The model under review builds one solid part; all positions refer to its coordinate system, in mm. Face numbers are marked on the shaded views. A direction names the side the tool comes from. Give positions to 0.01 mm unless a question says otherwise; leave off trailing zeros. Order: outer loops, then holes, each group sorted by start corner. A loop starts at its lowest first (then second) coordinate and runs counter-clockwise, first axis right, second up. Notation, with made-up numbers: (87, 59) - (132, 59) arc R22 cw to (132, 92) - close; hole circle Ø3 at (7.25, -21). An arc over 180 degrees is marked (long way). Put each result on its own line as item: value.
```python
from build123d import *
from build123d.topology import SkipClean

# Parameters (mm, degrees)
SKETCH1_R           = 1
SKETCH1_R_2         = 0.9
BOSS_EXTRUDE1_DEPTH = 10
SKETCH2_R           = 1
SKETCH2_R_2         = 0.9
BOSS_EXTRUDE2_DEPTH = 5
SKETCH4_R           = 0.9
CUT_EXTRUDE2_DEPTH  = 12.224972294
SKETCH5_R           = 0.9
CUT_EXTRUDE3_DEPTH  = 15.17744702


with BuildPart() as part:
    # Sketch1 → Boss-Extrude1 (new body)
    with BuildSketch(Plane(origin=(0, 0, 0), x_dir=(1, 0, 0), z_dir=(0, 1, 0))):
        with Locations(Location((0, 0, 0), (0, 0, 270))):
            Circle(SKETCH1_R)
        with Locations(Location((0, 0, 0), (0, 0, 270))):
            Circle(SKETCH1_R_2, mode=Mode.SUBTRACT)
    extrude(amount=BOSS_EXTRUDE1_DEPTH)

    # Sketch2 → Boss-Extrude2 (add, symmetric)
    with BuildSketch(Plane(origin=(0, 0, 0), x_dir=(0, 0, -1), z_dir=(1, 0, 0))):
        with Locations((0, 5)):
            Circle(SKETCH2_R)
        with Locations(Location((0, 5, 0), (0, 0, 180))):
            Circle(SKETCH2_R_2, mode=Mode.SUBTRACT)
    extrude(amount=BOSS_EXTRUDE2_DEPTH, both=True)

    # Sketch4 → Cut-Extrude2 (cut, through all)
    with BuildSketch(Plane.XZ):
        with Locations(Location((0, 0, 0), (0, 0, 90))):
            Circle(SKETCH4_R)
    extrude(amount=-CUT_EXTRUDE2_DEPTH, mode=Mode.SUBTRACT)

    # Sketch5 → Cut-Extrude3 (cut, through all)
    with SkipClean():  # the faces are left unmerged after this step: merging them gives an invalid solid
        with BuildSketch(Plane(origin=(5, 0, 0), x_dir=(0, 0, -1), z_dir=(1, 0, 0))):
            with Locations((0, 5)):
                Circle(SKETCH5_R)
        extrude(amount=-CUT_EXTRUDE3_DEPTH, mode=Mode.SUBTRACT)


solid = part.part
```
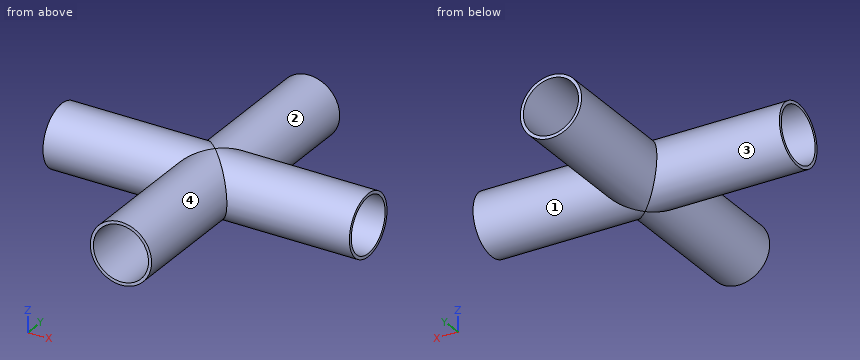
(1) The part is to be moulded in two halves that separate along Y. For the marked faces 1 and 2, say which applies: pulls with the +Y half, pulls with the -Y half, needs draft (parallel to the pull), parting line crosses it, or undercut.
The answers:
face 1: parting line crosses it
face 2: needs draft
(2) Take a section at D-D, the plane x = -3.25. Write out the cut boundary in (y, z), then the cut area to 3 significant figures.
The answers:
outline: circle Ø2 at (5, 0); hole circle Ø1.8 at (5, 0)
area: 0.597 mm^2
(3) Take a section at A-A, the plane z = 0. Write out the cut boundary in (x, y).
The answers:
outline: (-5, 4) - (-1, 4) - (-1, 0) - (-0.9, 0) - (-0.9, 4.1) - (-5, 4.1) - close; (-5, 5.9) - (-0.9, 5.9) - (-0.9, 10) - (-1, 10) - (-1, 6) - (-5, 6) - close; (0.9, 0) - (1, 0) - (1, 4) - (5, 4) - (5, 4.1) - (0.9, 4.1) - close; (0.9, 5.9) - (5, 5.9) - (5, 6) - (1, 6) - (1, 10) - (0.9, 10) - close
(4) Take a section at B-B, the plane y = 8.5. Write out the cut boundary in (x, z), then the cut area to 3 significant figures.
The answers:
outline: circle Ø2 at (0, 0); hole circle Ø1.8 at (0, 0)
area: 0.597 mm^2
(5) Clearance check with a flat-ended pin moving along its axis: pin 1 Ø2 at (x, y) = (-3.5, 8.5) entering from -Z. State where the tip first meets the part, or that it passes through.
The answers:
pin 1: through
(6) Wall thickness on L1, parallel to Y at x = -0.5, z = 0.8: over which ranges is the line inside the solid? List them lowest first.
The answers:
L1: 0 to 4.59, 5.41 to 10
(7) For the marked faces 3 and 4, list the 3-axis set-ups (+Z, -Z, +X, -X, +Y, -Y) from which the entire face can be reached by the end or side of a thin tool; tool diameter is ignored.
The answers:
face 3: -X
face 4: -Y
(8) Take a section at C-C, the plane x = 0.75. Write out the cut boundary in (y, z).
The answers:
outline: (0, -0.66) - (4.25, -0.66) arc R1 ccw to (5.75, -0.66) - (10, -0.66) - (10, -0.5) - (5.75, -0.5) arc R0.9 cw to (4.25, -0.5) - (0, -0.5) - close; (0, 0.5) - (4.25, 0.5) arc R0.9 cw to (5.75, 0.5) - (10, 0.5) - (10, 0.66) - (5.75, 0.66) arc R1 ccw to (4.25, 0.66) - (0, 0.66) - close
